Read the model definition and answer for the solid it produces. Units are mm, in the model's axes. A direction names the side the tool comes from. Coordinates: 2 decimals unless noted, no trailing zeros. Write each loop counter-clockwise with the first axis right and the second up, starting at its lowest first coordinate (ties: lowest second). Pieces come first, ordered by that corner, then holes.
(1) The part is cut by section A-A, the plane z = 2. Determine the outline of the cut face in (x, y), and give its area (3 significant figures).
(2) The part is cut by section C-C, the plane x = -14.5. Determine the outline of the cut face in (y, z), and give its area (3 significant figures).
(3) The part is cut by section B-B, the plane x = -37.5. Determine the outline of the cut face in (y, z), and give its area (3 significant figures).
(4) The part is cut by section D-D, the plane x = 37.5. Determine the outline of the cut face in (y, z).
(5) Determine the mould class of faces 6 (the cylindrical face through (-38.538, 7.888, -18.004)), 7 (the flat face through (41, 8, -8.25)), 8 (the flat face through (45, 13, 0)) for opening direction X: pulls with the +X half, pulls with the -X half, needs draft (parallel to the pull), parting line crosses it, or undercut.
(6) Which of the six approach directions +Z, -Z, +X, -X, +Y, -Y give full straight-line access (tool end or side, diameter ignored) to faces 1 (the flat face through (-43, 1.75, 15)), 2 (the flat face through (30, 8, 20)), 3 (the flat face through (43, 3.75, 0)), 4 (the flat face through (42, 7.9, 24.5)), 5 (the flat face through (-1, 8, 27.5))?
(7) Given pin 1 (8 mm diameter, centred on y = 7.5, z = 4.5, fed in from -X); pin 2 (1.6 mm diameter, centred on y = 7.5, z = -10, fed in from +X); pin 3 (1.2 mm diameter, centred on x = -43, y = 8.5, fed in from +Z), each flat-ended and moving along its own axis, determine where each tip first touches the part or whether it passes through.
(8) Straight lines are drawn through the part: line 1 along X through (y, z) = (7.5, -20); line 2 along Z through (x, y) = (-37.5, 7.5); line 3 along Z through (x, y) = (37.5, 7). For each, find the intervals that lie inside material, in ascending order.
```python
from build123d import *

# Parameters (mm, degrees)
SKETCH1_W            = 90
SKETCH1_H            = 55
BOSS_EXTRUDE1_DEPTH  = 16
SKETCH2_W            = 22
SKETCH2_H            = 1.75
SKETCH2_H_2          = 12.5
CUT_EXTRUDE1_DEPTH   = 4
SKETCH3_W            = 20
SKETCH3_H            = 13
CUT_EXTRUDE2_DEPTH   = 20
CHAMFER1_SIZE        = 6
M4_CLEARANCE_HOLE1_D = 4.5
SKETCH7_W            = 27.5
SKETCH7_H            = 8.5
CUT_EXTRUDE3_DEPTH   = 3
SKETCH8_W            = 16.5
SKETCH8_H            = 8.5
CUT_EXTRUDE4_DEPTH   = 12
SKETCH9_R            = 2.25
CUT_EXTRUDE5_DEPTH   = 17
CHAMFER2_SIZE        = 5


with BuildPart() as part:
    # Sketch1 → Boss-Extrude1 (new body)
    with BuildSketch(Plane(origin=(0, 0, 0), x_dir=(1, 0, 0), z_dir=(0, 1, 0))):
        Rectangle(SKETCH1_W, SKETCH1_H)
    extrude(amount=BOSS_EXTRUDE1_DEPTH)

    # Sketch2 → Cut-Extrude1 (cut)
    with BuildSketch(Plane.ZY.offset(45)):
        with Locations((0, 15.125)):
            Rectangle(SKETCH2_W, SKETCH2_H)
        Polygon((11, 16), (11, 14.25), (13, 14.25), (11.25, 16), align=None)
        Polygon((-11.25, 16), (-13, 14.25), (-11, 14.25), (-11, 16), align=None)
        Polygon((-17.5, 14.25), (-17.5, 1.75), (-13, 1.75), (-11, 1.75), (-11, 14.25), (-13, 14.25), align=None)
        with Locations((0, 8)):
            Rectangle(SKETCH2_W, SKETCH2_H_2)
        Polygon((11, 14.25), (11, 1.75), (13, 1.75), (17.5, 1.75), (17.5, 14.25), (13, 14.25), align=None)
        with Locations((0, 0.875)):
            Rectangle(SKETCH2_W, SKETCH2_H)
        Polygon((13, 1.75), (11, 1.75), (11, 0), (11.25, 0), align=None)
        Polygon((-11, 1.75), (-13, 1.75), (-11.25, 0), (-11, 0), align=None)
    extrude(amount=-CUT_EXTRUDE1_DEPTH, mode=Mode.SUBTRACT)

    # Sketch3 → Cut-Extrude2 (cut)
    with BuildSketch(Plane.ZY.offset(41)):
        with Locations((0, 8)):
            Rectangle(SKETCH3_W, SKETCH3_H)
    extrude(amount=-CUT_EXTRUDE2_DEPTH, mode=Mode.SUBTRACT)

    # Chamfer1
    chamfer1_edges = [part.edges().sort_by_distance(p)[0] for p in [
        (45, 8, 27.5),
        (-45, 8, 27.5),
        (-45, 8, -27.5),
        (45, 8, -27.5),
    ]]
    chamfer(chamfer1_edges, length=CHAMFER1_SIZE)

    # M4 Clearance Hole1 (through all)
    with Locations(Plane(origin=(0, 16, 0), x_dir=(1, 0, 0), z_dir=(0, 1, 0))):
        with Locations((0, 0), (37.5, 20), (-37.5, -20), (-37.5, 20), (37.5, -20)):
            Hole(M4_CLEARANCE_HOLE1_D / 2)

    # Sketch7 → Cut-Extrude3 (cut)
    with BuildSketch(Plane(origin=(45, 0, 0), x_dir=(0, 0, -1), z_dir=(1, 0, 0))):
        with Locations((0, 8)):
            Rectangle(SKETCH7_W, SKETCH7_H)
    extrude(amount=-CUT_EXTRUDE3_DEPTH, mode=Mode.SUBTRACT)

    # Sketch8 → Cut-Extrude4 (cut)
    with BuildSketch(Plane(origin=(42, 0, 0), x_dir=(0, 0, -1), z_dir=(1, 0, 0))):
        with Locations((0, 8)):
            Rectangle(SKETCH8_W, SKETCH8_H)
    extrude(amount=-CUT_EXTRUDE4_DEPTH, mode=Mode.SUBTRACT)

    # Sketch9 → Cut-Extrude5 (cut, through all)
    with BuildSketch(Plane(origin=(0, 16, 0), x_dir=(1, 0, 0), z_dir=(0, 1, 0))):
        Polygon((30, -12.5), (40, -12.5), (40, 12.5), (30, 12.5), (30, 22.5), (-30, 22.5), (-30, 12.5), (-36, 12.5), (-36, -12.5), (-30, -12.5), (-30, -22.5), (30, -22.5), align=None)
        Circle(SKETCH9_R, mode=Mode.SUBTRACT)
    extrude(amount=-CUT_EXTRUDE5_DEPTH, mode=Mode.SUBTRACT)

    # Chamfer2
    chamfer2_edges = [part.edges().sort_by_distance(p)[0] for p in [
        (30, 8, -12.5),
        (30, 8, 12.5),
        (-30, 8, 12.5),
        (-30, 8, -12.5),
    ]]
    chamfer(chamfer2_edges, length=CHAMFER2_SIZE)


solid = part.part
```
Computed:
1. outline: (-41, 0) - (-36, 0) - (-36, 1.5) - (-41, 1.5) - close; (-41, 14.5) - (-36, 14.5) - (-36, 16) - (-41, 16) - close; (40, 0) - (45, 0) - (45, 3.75) - (40, 3.75) - close; (40, 12.25) - (45, 12.25) - (45, 16) - (40, 16) - close
1. area: 52.5 mm2
2. outline: (0, -27.5) - (16, -27.5) - (16, -22.5) - (0, -22.5) - close; (0, 22.5) - (16, 22.5) - (16, 27.5) - (0, 27.5) - close
2. area: 160 mm2
3. outline: (0, -27.5) - (16, -27.5) - (16, -22.25) - (0, -22.25) - close; (0, -17.75) - (16, -17.75) - (16, 17.75) - (0, 17.75) - close; (0, 22.25) - (16, 22.25) - (16, 27.5) - (0, 27.5) - close; hole (1.5, -10) - (14.5, -10) - (14.5, 10) - (1.5, 10) - close
3. area: 476 mm2
4. outline: (0, -27.5) - (16, -27.5) - (16, -22.25) - (0, -22.25) - close; (0, -17.75) - (16, -17.75) - (16, -12.5) - (0, -12.5) - close; (0, 12.5) - (16, 12.5) - (16, 17.75) - (0, 17.75) - close; (0, 22.25) - (16, 22.25) - (16, 27.5) - (0, 27.5) - close
5. face 6: undercut
5. face 7: needs draft
5. face 8: pulls with the +X half
6. face 1: -X
6. face 2: +Y, -Y
6. face 3: +X
6. face 4: +Z, +X, +Y, -Y
6. face 5: +Z, +X, -X, +Y, -Y
7. pin 1: stops at x = 40
7. pin 2: stops at x = 42
7. pin 3: stops at z = 24.1
8. line 1: x = -45 to -39.75, -35.25 to -30, 30 to 35.25, 39.75 to 45
8. line 2: z = -27.5 to -22.25, -17.75 to -10, 10 to 17.75, 22.25 to 27.5
8. line 3: z = -27.5 to -22.25, -17.75 to -12.5, 12.5 to 17.75, 22.25 to 27.5
